For this review, take the finished solid that the model builds, in its own axes (mm). Round coordinates to 2 decimals unless told otherwise and drop trailing zeros. Write each loop counter-clockwise with the first axis right and the second up, starting at its lowest first coordinate (ties: lowest second). Pieces come first, ordered by that corner, then holes. Notation, with made-up numbers: (-26, 9) -> (-13, 9) arc R30 ccw to (-13, 41) -> close; hole circle Ø11 at (64, -9). An arc over 180 degrees is marked (long way). Write each question's results on one line, items separated by ' | '. Start each with the question number.
Item 1: The part is to be moulded in two halves that separate along X. For faces 1 (the cylindrical face through (-2.03, 0.04, 1.05)), 2 (the flat face through (91, 3.175, 0)), 3 (the cylindrical face through (184.15, -0.76, -0.1)), say which applies: +X half, -X half, draft (parallel to the pull), parting line (faces both ways), or undercut.
Item 2: Add section C-C (y = -1.25). State the section outline as (x, z) points (1 decimal), plus the area to 3 significant figures.
Item 3: To check wall thickness, follow line 1 along X through (y, z) = (-1.5, 0); line 2 along X through (y, z) = (0, 1.25); line 3 along Y through (x, z) = (84, 3.25) (3 decimals). State the ranges of each line that lie inside material, in increasing order.
Item 4: Add section A-A (z = 0). Count the separate pieces of the cut face and the enclosed holes in it, plus the area to 3 significant figures.
Item 5: Add section B-B (x = 160). State the section outline as (y, z) points (1 decimal), plus the area to 3 significant figures.
from build123d import *

# Parameters (mm, degrees)
BOSS_EXTRUDE1_DEPTH = 3.175
SKETCH2_R           = 2.286
CUT_EXTRUDE1_DEPTH  = 185.320987428
FILLET1_R           = 1.5875


with BuildPart() as part:
    # Sketch1 → Boss-Extrude1 (new, symmetric)
    with BuildSketch(Plane(origin=(0, 0, 0), x_dir=(1, 0, 0), z_dir=(0, 1, 0))):
        with BuildLine():
            Line((0, 4.7625), (179.3875, 4.7625))
            ThreePointArc((179.3875, 4.7625), (184.15, 0), (179.3875, -4.7625))
            Line((179.3875, -4.7625), (0, -4.7625))
            ThreePointArc((0, -4.7625), (-4.7625, 0), (0, 4.7625))
        make_face()
    extrude(amount=BOSS_EXTRUDE1_DEPTH, both=True)

    # Sketch2 → Cut-Extrude1 (cut, through all)
    with BuildSketch(Plane(origin=(0, 3.175, 0), x_dir=(1, 0, 0), z_dir=(0, 1, 0))):
        with Locations(Location((0, 0, 0), (0, 0, 270))):
            Circle(SKETCH2_R)
        with Locations(Location((179.3875, 0, 0), (0, 0, 270))):
            Circle(SKETCH2_R)
    extrude(amount=-CUT_EXTRUDE1_DEPTH, mode=Mode.SUBTRACT)

    # Fillet1
    fillet1_edges = [part.edges().sort_by_distance(p)[0] for p in [
        (184.15, 3.175, 0),
        (89.69375, 3.175, -4.7625),
        (-4.7625, 3.175, 0),
        (89.69375, 3.175, 4.7625),
    ]]
    fillet(fillet1_edges, radius=FILLET1_R)


solid = part.part
Responses:
1) face 1: undercut | face 2: draft | face 3: +X half
2) outline: (0, -4.8) -> (179.4, -4.8) arc R4.8 ccw to (179.4, 4.8) -> (0, 4.8) arc R4.8 ccw to start; hole circle Ø4.6 at (0, 0); hole circle Ø4.6 at (179.4, 0) | area: 1,750 mm^2
3) line 1: x = -4.76 to -2.29, 2.29 to 177.1, 181.67 to 184.15 | line 2: x = -4.6 to -1.91, 1.91 to 177.47, 181.3 to 183.98 | line 3: y = -3.175 to 3.173
4) separate pieces: 3 | enclosed holes: 0 | area: 1,140 mm^2
5) outline: (-3.2, -4.8) -> (1.6, -4.8) arc R1.6 ccw to (3.2, -3.2) -> (3.2, 3.2) arc R1.6 ccw to (1.6, 4.8) -> (-3.2, 4.8) -> close | area: 59.4 mm^2
